For this review, take the finished solid that the model builds, in its own axes (mm). Face numbers are marked on the shaded views. A direction names the side the tool comes from. Give positions to 0.01 mm unless a question says otherwise; leave off trailing zeros. Loops run counter-clockwise (first coordinate to the right, second up) from the corner with the lowest first, then second, coordinate; pieces in that order, holes last. Notation, with made-up numbers: (24.25, -38.5) -> (37.25, -38.5) arc R24 ccw to (37.25, -25.5) -> close; hole circle Ø3 at (-19, 1). An arc over 180 degrees is marked (long way). Answer as CSV lines item,"result". Start each with the question number.
Item 1: Clearance check with flat-ended pins moving along their axes: P1, Ø1, axis at y = 16, z = 24, coming from the -X side; P2, Ø4, axis at x = -7.5, z = 26.5, coming from the -Y side; P3, Ø3, axis at y = 8.5, z = 26.5, coming from the +X side. State where each tip first meets the part, or that it passes through.
Item 2: Machinability: for the marked faces 1 and 2, which of the approach directions +Z, -Z, +X, -X, +Y, -Y give a long, thin tool a straight path to every point of the face, cutting with its end or side? Answer none if there is none.
Item 3: For L1, parallel to X at y = -8, z = 11.5; L2, parallel to X at y = 0.5, z = 26.5; L3, parallel to X at y = -9, z = 20.5, list the stretches that pass through material, from the lowest coordinate up. Write a range as from..to.
Item 4: Add section A-A on x = 0. State the section outline as (y, z) points.
Item 5: Add section B-B on z = 20.75. State how many separate pieces and enclosed holes the cut face has, plus the area to 3 significant figures.
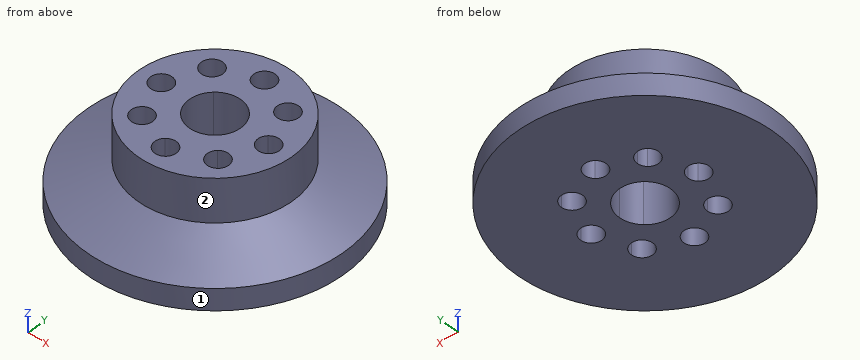
```python
from build123d import *

# Parameters (mm, degrees)
F0_R     = 30
F1_DEPTH = 20
F2_SIZE2 = 5
F2_SIZE  = 12
F3_DEPTH = 20
F5_DEPTH = 50
F6_DEPTH = 10
F7_DEPTH = 10


with BuildPart() as f1:
    # F0 (on Top) → F1 (new body)
    with BuildSketch(Plane.XY):
        Circle(F0_R)
    extrude(amount=F1_DEPTH)

    # F2
    f2_edges = [f1.edges().sort_by_distance(p)[0] for p in [
        (-30, 0, 20),
    ]]
    f2_side = f1.faces().sort_by_distance((0, 0, 20))[0]
    chamfer(f2_edges, length=F2_SIZE, length2=F2_SIZE2, reference=f2_side)

    # F3 (add): a face of the model
    f3_faces = [f1.faces().sort_by_distance(p)[0] for p in [
        (0, 0, 20),
    ]]
    extrude(f3_faces, amount=F3_DEPTH)

    # F4 (on face) → F5 (cut)
    with BuildSketch(Plane.XY.offset(40)):
        with BuildLine():
            Line((-12.73, 0), (-10.962233047, 1.767766953))
            ThreePointArc((-10.962233047, 1.767766953), (-15.23, 0), (-10.962233047, -1.767766953))
            Line((-10.962233047, -1.767766953), (-12.73, 0))
        make_face()
        with BuildLine():
            ThreePointArc((-10.23, 0), (-10.4203011687, 0.9567085809), (-10.962233047, 1.767766953))
            Line((-10.962233047, 1.767766953), (-12.73, 0))
            Line((-12.73, 0), (-10.962233047, -1.767766953))
            ThreePointArc((-10.962233047, -1.767766953), (-10.4203011687, -0.9567085809), (-10.23, 0))
        make_face()
        with BuildLine():
            Line((0, 0), (4.2426406871, 4.2426406871))
            ThreePointArc((4.2426406871, 4.2426406871), (0, 6), (-4.2426406871, 4.2426406871))
            Line((-4.2426406871, 4.2426406871), (0, 0))
        make_face()
        with BuildLine():
            Line((0, 0), (-4.2426406871, 4.2426406871))
            ThreePointArc((-4.2426406871, 4.2426406871), (-6, 0), (-4.2426406871, -4.2426406871))
            Line((-4.2426406871, -4.2426406871), (0, 0))
        make_face()
        with BuildLine():
            ThreePointArc((-4.2426406871, -4.2426406871), (0, -6), (4.2426406871, -4.2426406871))
            Line((4.2426406871, -4.2426406871), (0, 0))
            Line((0, 0), (-4.2426406871, -4.2426406871))
        make_face()
        with BuildLine():
            ThreePointArc((4.2426406871, -4.2426406871), (5.5432771951, -2.2961005942), (6, 0))
            ThreePointArc((6, 0), (5.5432771951, 2.2961005942), (4.2426406871, 4.2426406871))
            Line((4.2426406871, 4.2426406871), (0, 0))
            Line((0, 0), (4.2426406871, -4.2426406871))
        make_face()
        with BuildLine():
            ThreePointArc((-1.767766953, 10.962233047), (0, 10.23), (1.767766953, 10.962233047))
            Line((1.767766953, 10.962233047), (0, 12.73))
            Line((0, 12.73), (-1.767766953, 10.962233047))
        make_face()
        with BuildLine():
            Line((0, 12.73), (1.767766953, 10.962233047))
            ThreePointArc((1.767766953, 10.962233047), (2.3096988313, 11.7732914191), (2.5, 12.73))
            ThreePointArc((2.5, 12.73), (-0.9567085809, 15.0396988313), (-1.767766953, 10.962233047))
            Line((-1.767766953, 10.962233047), (0, 12.73))
        make_face()
        with BuildLine():
            Line((12.73, 0), (10.962233047, 1.767766953))
            ThreePointArc((10.962233047, 1.767766953), (10.23, 0), (10.962233047, -1.767766953))
            Line((10.962233047, -1.767766953), (12.73, 0))
        make_face()
        with BuildLine():
            ThreePointArc((15.23, 0), (13.6867085809, 2.3096988313), (10.962233047, 1.767766953))
            Line((10.962233047, 1.767766953), (12.73, 0))
            Line((12.73, 0), (10.962233047, -1.767766953))
            ThreePointArc((10.962233047, -1.767766953), (13.6867085809, -2.3096988313), (15.23, 0))
        make_face()
        with BuildLine():
            Line((0, -12.73), (1.767766953, -10.962233047))
            ThreePointArc((1.767766953, -10.962233047), (0, -10.23), (-1.767766953, -10.962233047))
            Line((-1.767766953, -10.962233047), (0, -12.73))
        make_face()
        with BuildLine():
            ThreePointArc((2.5, -12.73), (2.3096988313, -11.7732914191), (1.767766953, -10.962233047))
            Line((1.767766953, -10.962233047), (0, -12.73))
            Line((0, -12.73), (-1.767766953, -10.962233047))
            ThreePointArc((-1.767766953, -10.962233047), (-0.9567085809, -15.0396988313), (2.5, -12.73))
        make_face()
        with BuildLine():
            ThreePointArc((11.5014693245, 9.0014693245), (8.0447607436, 11.3111681558), (7.2337023715, 7.2337023715))
            ThreePointArc((7.2337023715, 7.2337023715), (9.9581779054, 6.6917704932), (11.5014693245, 9.0014693245))
        make_face()
        with BuildLine():
            ThreePointArc((-6.5014693245, 9.0014693245), (-11.3111681558, 9.9581779054), (-7.2337023715, 7.2337023715))
            ThreePointArc((-7.2337023715, 7.2337023715), (-6.6917704932, 8.0447607436), (-6.5014693245, 9.0014693245))
        make_face()
        with BuildLine():
            ThreePointArc((-6.5014693245, -9.0014693245), (-6.6917704932, -8.0447607436), (-7.2337023715, -7.2337023715))
            ThreePointArc((-7.2337023715, -7.2337023715), (-11.3111681558, -9.9581779054), (-6.5014693245, -9.0014693245))
        make_face()
        with BuildLine():
            ThreePointArc((11.5014693245, -9.0014693245), (9.9581779054, -6.6917704932), (7.2337023715, -7.2337023715))
            ThreePointArc((7.2337023715, -7.2337023715), (8.0447607436, -11.3111681558), (11.5014693245, -9.0014693245))
        make_face()
    extrude(amount=-F5_DEPTH, mode=Mode.SUBTRACT)

    # F6 (cut): a face of the model
    f6_faces = [f1.faces().sort_by_distance(p)[0] for p in [
        (-17.4908831175, 0, 40),
    ]]
    extrude(f6_faces, amount=-F6_DEPTH, mode=Mode.SUBTRACT)

    # F7 (cut): a face of the model
    f7_faces = [f1.faces().sort_by_distance(p)[0] for p in [
        (-29.1514718626, 0, 0),
    ]]
    extrude(f7_faces, amount=-F7_DEPTH, mode=Mode.SUBTRACT)


solid = f1.part
```
Computed values:
1,P1,"x = -9.15"
1,P2,"y = -17.14"
1,P3,"x = 16.58"
2,face 1,"+Z, -Z"
2,face 2,"+Z"
3,L1,"-28.91..-11.29, -6.71..6.71, 11.29..28.91"
3,L2,"-17.99..-15.18, -10.28..-5.98, 5.98..10.28, 15.18..17.99"
3,L3,"-15.59..-11.5, -6.5..6.5, 11.5..15.59"
4,outline,"(-30, 10) -> (-15.23, 10) -> (-15.23, 30) -> (-18, 30) -> (-18, 20) -> (-30, 15) -> close; (-10.23, 10) -> (-6, 10) -> (-6, 30) -> (-10.23, 30) -> close; (6, 10) -> (10.23, 10) -> (10.23, 30) -> (6, 30) -> close; (15.23, 10) -> (30, 10) -> (30, 15) -> (18, 20) -> (18, 30) -> (15.23, 30) -> close"
5,separate pieces,"1"
5,enclosed holes,"9"
5,area,"748 mm²"
